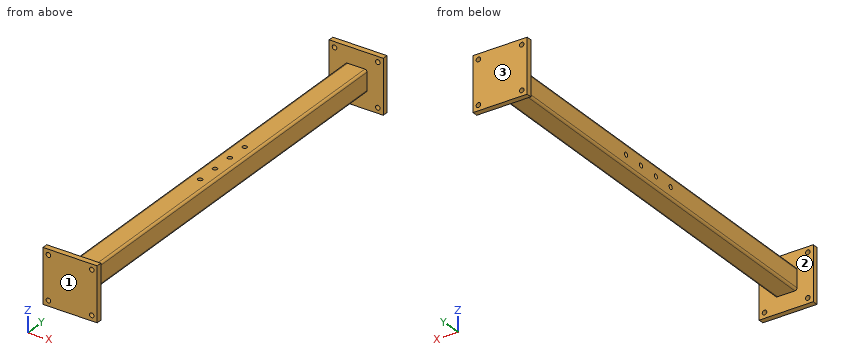
from build123d import *

# Parameters (mm, degrees)
F0_W           = 50.8
F0_H           = 50.8
F1_DEPTH       = 482.6
F2_W           = 127
F2_H           = 127
F2_W_2         = 50.8
F2_H_2         = 50.8
F3_DEPTH       = 12.7
F4_R           = 5.08
F5_D           = 10.71626
F9_D           = 10.71626
F9_DEPTH       = 31.2615384615
F9_TIP         = 3.2194893086
F9_ON_F8_D     = 10.71626
F9_ON_F8_DEPTH = 31.2615384615
F9_ON_F8_TIP   = 3.2194893086


# Not quite as in the source:
# - a feature names something its author has since deleted; it is built from what else it names


with BuildPart() as f1:
    # F0 (on Front) → F1 (new body, symmetric)
    with BuildSketch(Plane.XZ):
        Rectangle(F0_W, F0_H)
    extrude(amount=F1_DEPTH, both=True)

    # F2 (on face) → F3 (join)
    with BuildSketch(Plane.XZ.offset(482.6)):
        Rectangle(F2_W, F2_H)
        Rectangle(F2_W_2, F2_H_2, mode=Mode.SUBTRACT)
        Rectangle(F2_W_2, F2_H_2)
    extrude(amount=F3_DEPTH)

    # F4
    f4_edges = [f1.edges().sort_by_distance(p)[0] for p in [
        (25.4, 0, 25.4),
        (-25.4, 0, 25.4),
        (-25.4, 0, -25.4),
        (25.4, 0, -25.4),
    ]]
    fillet(f4_edges, radius=F4_R)

    # F5 (through all)
    with Locations(Plane(origin=(0, -482.6, 0), x_dir=(1, 0, 0), z_dir=(0, 1, 0))):
        with Locations((-50.8, -50.8), (50.8, -50.8), (50.8, 50.8), (-50.8, 50.8)):
            Hole(F5_D / 2)

    # F6: F1 across plane


with BuildPart() as f1_1:
    add(f1.part)
    add(f1.part.mirror(Plane.XZ))

    # F9
    with Locations(Plane(origin=(-25.4, 0, 0), x_dir=(0, -1, 0), z_dir=(-1, 0, 0))):
        with Locations((-50.8, 0), (50.8, 0), (-101.6, 0), (0, 0)):
            Hole(F9_D / 2, depth=F9_DEPTH)
            with Locations((0, 0, -(F9_DEPTH + F9_TIP / 2))):  # 118° drill point
                Cone(0, F9_D / 2, F9_TIP, mode=Mode.SUBTRACT)

    # F9 on F8
    with Locations(Plane.XY.offset(25.4)):
        with Locations((0, 0), (0, 101.6), (0, 50.8), (0, -50.8)):
            Hole(F9_ON_F8_D / 2, depth=F9_ON_F8_DEPTH)
            with Locations((0, 0, -(F9_ON_F8_DEPTH + F9_ON_F8_TIP / 2))):  # 118° drill point
                Cone(0, F9_ON_F8_D / 2, F9_ON_F8_TIP, mode=Mode.SUBTRACT)


solid = f1_1.part
Part model, mm, in its own coordinate system. Face numbers are marked on the shaded views. Coordinates: 2 decimals unless noted, no trailing zeros. Write each loop counter-clockwise with the first axis right and the second up, starting at its lowest first coordinate (ties: lowest second). Pieces come first, ordered by that corner, then holes. Notation, with made-up numbers: M 18,-30.75 L 62,-30.75 A35 cw 62,8.25 Z; hole C -3,46.5 d5. An arc over 180 degrees is marked long. Return JSON: item names as keys, results as strings.
1. Saw through at A-A, the plane y = 166.5. Write the cut outline in (x, z).
Determined:
{"outline": "M -25.4,-20.32 A5.08 ccw -20.32,-25.4 L 20.32,-25.4 A5.08 ccw 25.4,-20.32 L 25.4,20.32 A5.08 ccw 20.32,25.4 L -20.32,25.4 A5.08 ccw -25.4,20.32 Z"}
2. Pull direction Y, two halves, no side cores. Call the marked faces 1, 2 and 3: pulls with the +Y half, pulls with the -Y half, needs draft (parallel to the pull), parting line crosses it, or undercut.
Determined:
{"face 1": "pulls with the -Y half", "face 2": "undercut", "face 3": "pulls with the +Y half"}
3. Flat gauge pins, fed straight in: pin 1 Ø17 at (y, z) = (101.6, 0) entering from -X; pin 2 Ø17 at (x, y) = (0, 101.6) entering from -Z; pin 3 Ø5 at (y, z) = (252, 24.5) entering from +X. Where does each tip first touch, or does it go through?
Determined:
{"pin 1": "x = -25.4", "pin 2": "z = -25.4", "pin 3": "x = 25.11"}
4. Probe L1, parallel to Y at x = 0, z = -2; L2, parallel to X at y = 486.75, z = -50.8; L3, parallel to Y at x = 56.5, z = -35. List the from-to ranges inside material, lowest first.
Determined:
{"L1": "-495.3 to -56.16, -45.44 to -5.36, 5.36 to 45.44, 56.16 to 96.24, 106.96 to 495.3", "L2": "-63.5 to -56.16, -45.44 to 45.44, 56.16 to 63.5", "L3": "-495.3 to -482.6, 482.6 to 495.3"}
